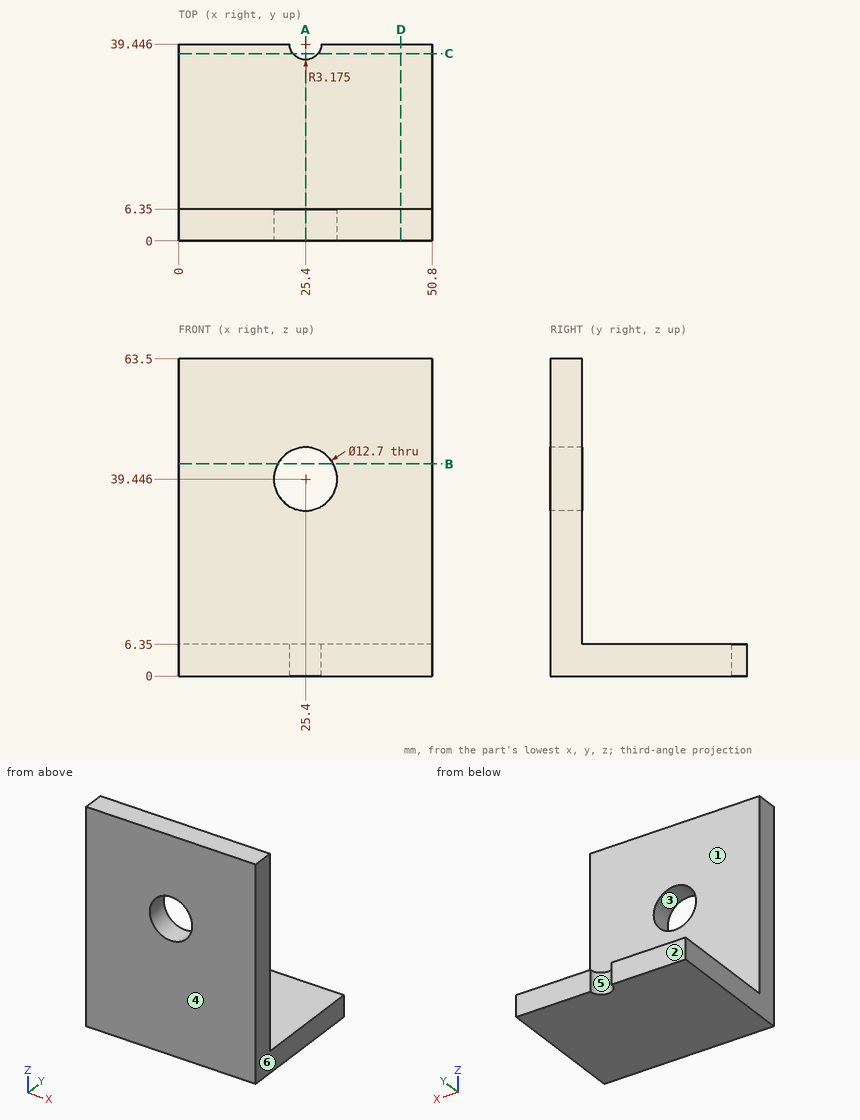
Source: three-view drawing plus pictorial views. Frame: mm from the lowest corner of the part. A direction names the side the tool comes from. Coordinates: 2 decimals unless noted, no trailing zeros. Write each loop counter-clockwise with the first axis right and the second up, starting at its lowest first coordinate (ties: lowest second). Pieces come first, ordered by that corner, then holes. Notation, with made-up numbers: (80.25, 17) - (117.25, 17) arc R36 cw to (117.25, 52) - close; hole circle Ø2 at (85, 42). An arc over 180 degrees is marked (long way). Answer as a JSON object with one key per item and string values.
Q1. Section query C-C, the plane y = 37.5. Output: boundary loops of the cut face in (x, z).
Ans:
{"outline": "(0, 0) - (22.89, 0) - (22.89, 6.35) - (0, 6.35) - close; (27.91, 0) - (50.8, 0) - (50.8, 6.35) - (27.91, 6.35) - close"}
Q2. Set-up query: the marked faces 1 and 2. Return all of +Z, -Z, +X, -X, +Y, -Y with unobstructed straight access to the full face (end or side cutting, diameter ignored); none if empty.
Ans:
{"face 1": "+Z, +X, -X, +Y", "face 2": "+Z, -Z, +X, -X, +Y"}
Q3. First-contact query: pin 1 Ø1 at (x, z) = (44.5, 8.5) entering from +Y; pin 2 Ø5 at (x, y) = (44.5, 19) entering from -Z. Flat tips, straight axial feed; report the tip coordinate or a pass-through.
Ans:
{"pin 1": "stops at y = 6.35", "pin 2": "stops at z = 0"}
Q4. Draft query along X for the marked faces 3, 4, 5 and 6. Return one class per face: released by +X, released by -X, zero draft, split by the parting line, or undercut.
Ans:
{"face 3": "undercut", "face 4": "zero draft", "face 5": "undercut", "face 6": "released by +X"}
Q5. Material intervals for line 1 (Z direction, x = 25, y = 1); line 2 (Y direction, x = 36, z = 31), sorted ascending. Write a range as [from, to].
Ans:
{"line 1": "z = [0, 33.11], [45.78, 63.5]", "line 2": "y = [0, 6.35]"}
Q6. Section query B-B, the plane z = 42.5. Output: boundary loops of the cut face in (x, y).
Ans:
{"outline": "(0, 0) - (19.83, 0) - (19.83, 6.35) - (0, 6.35) - close; (30.97, 0) - (50.8, 0) - (50.8, 6.35) - (30.97, 6.35) - close"}
Q7. Section query D-D, the plane x = 44.5. Output: boundary loops of the cut face in (y, z), plus the area to 3 significant figures.
Ans:
{"outline": "(0, 0) - (39.45, 0) - (39.45, 6.35) - (6.35, 6.35) - (6.35, 63.5) - (0, 63.5) - close", "area": "613 mm2"}
Q8. Section query A-A, the plane x = 25.4. Output: boundary loops of the cut face in (y, z).
Ans:
{"outline": "(0, 0) - (36.27, 0) - (36.27, 6.35) - (6.35, 6.35) - (6.35, 33.1) - (0, 33.1) - close; (0, 45.8) - (6.35, 45.8) - (6.35, 63.5) - (0, 63.5) - close"}
